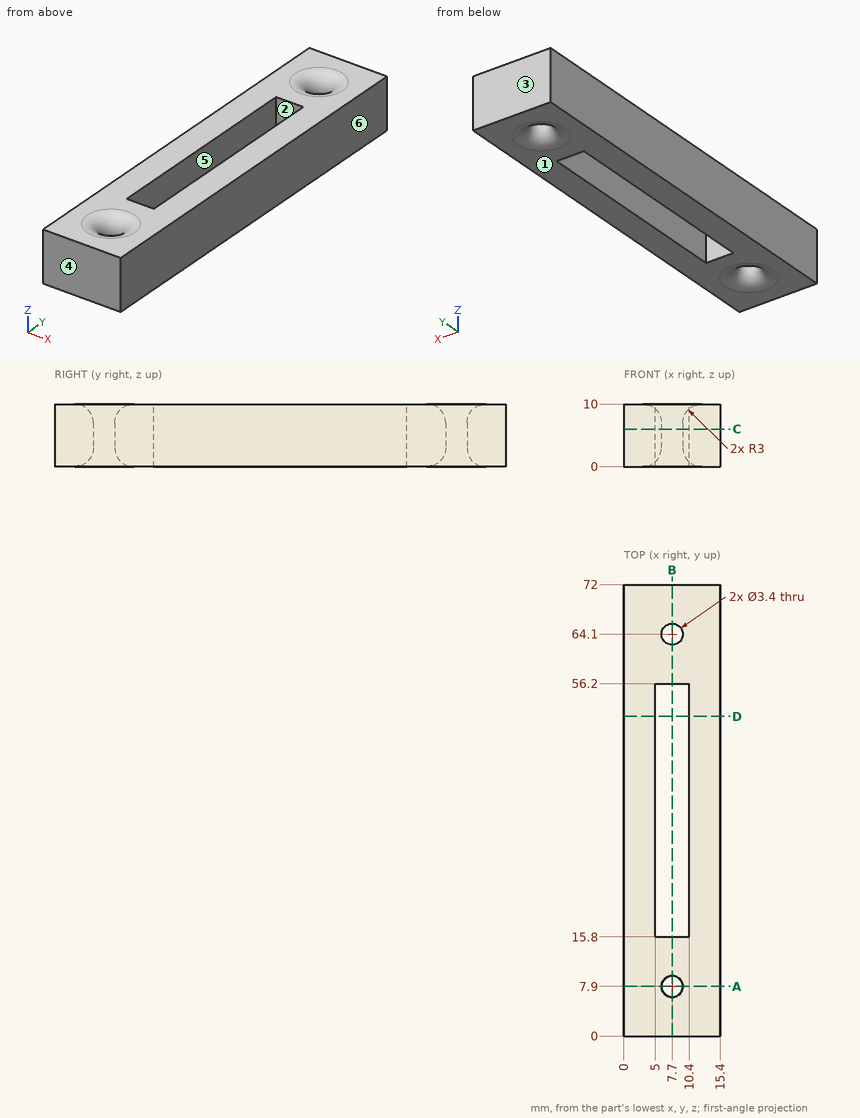
Design review of the part shown in the three views and the two pictorial views. Dimensions are in mm from the part's minimum x, y and z. A direction names the side the tool comes from. Give positions to 0.01 mm unless a question says otherwise; leave off trailing zeros. Loops run counter-clockwise (first coordinate to the right, second up) from the corner with the lowest first, then second, coordinate; pieces in that order, holes last. Notation, with made-up numbers: (67.25, -25) -> (102.25, -25) arc R16 ccw to (102.25, -1) -> close; hole circle Ø3 at (88, 71). An arc over 180 degrees is marked (long way). Answer as a JSON object with one key per item and string values. Group by question number.
Q1. Draft analysis for pull direction Y (two halves, no side actions). For the marked faces 1, 2, 3 and 4, state which applies: pulls with the +Y half, pulls with the -Y half, needs draft (parallel to the pull), parting line crosses it, or undercut.
Q2. Wall thickness on line 1 along Y through (x, z) = (7.7, 5.25); line 2 along X through (y, z) = (52, 7.25); line 3 along Y through (x, z) = (6.5, 1): over which ranges is each line inside the solid? List them lowest first.
Q3. Take a section at A-A (y = 7.9). Write out the cut boundary in (x, z), plus the area to 3 significant figures.
Q4. Take a section at C-C (z = 6). Write out the cut boundary in (x, y), plus the area to 3 significant figures.
Q5. Take a section at B-B (x = 7.7). Write out the cut boundary in (y, z).
Q6. Insertion check: pin 1 (4.5 mm diameter, centred on x = 7.7, y = 64.1, fed in from +Z); pin 2 (3 mm diameter, centred on x = 7.7, y = 7.9, fed in from -Z). Each pin has a flat end and moves straight along its axis. Give the tip position at first contact, or say it passes through.
Q7. Take a section at D-D (y = 51). Write out the cut boundary in (x, z).
Q8. Tool access review of the marked faces 5 and 6: name each direction out of +Z, -Z, +X, -X, +Y, -Y from which nothing blocks a thin tool from reaching the whole face with its end or side.
Answer below:
{
 "1": {"face 1": "needs draft", "face 2": "undercut", "face 3": "pulls with the +Y half", "face 4": "pulls with the -Y half"},
 "2": {"line 1": "y = 0 to 6.2, 9.6 to 15.8, 56.2 to 62.4, 65.8 to 72", "line 2": "x = 0 to 5, 10.4 to 15.4", "line 3": "y = 0 to 5.75, 10.05 to 15.8, 56.2 to 61.95, 66.25 to 72"},
 "3": {"outline": "(0, 0) -> (3, 0) arc R3 ccw to (6, 3) -> (6, 7) arc R3 ccw to (3, 10) -> (0, 10) -> close; (9.4, 3) arc R3 ccw to (12.4, 0) -> (15.4, 0) -> (15.4, 10) -> (12.4, 10) arc R3 ccw to (9.4, 7) -> close", "area": "112 mm2"},
 "4": {"outline": "(0, 0) -> (15.4, 0) -> (15.4, 72) -> (0, 72) -> close; hole (5, 15.8) -> (10.4, 15.8) -> (10.4, 56.2) -> (5, 56.2) -> close; hole circle Ø3.4 at (7.7, 7.9); hole circle Ø3.4 at (7.7, 64.1)", "area": "872 mm2"},
 "5": {"outline": "(0, 0) -> (3.2, 0) arc R3 ccw to (6.2, 3) -> (6.2, 7) arc R3 ccw to (3.2, 10) -> (0, 10) -> close; (9.6, 3) arc R3 ccw to (12.6, 0) -> (15.8, 0) -> (15.8, 10) -> (12.6, 10) arc R3 ccw to (9.6, 7) -> close; (56.2, 0) -> (59.4, 0) arc R3 ccw to (62.4, 3) -> (62.4, 7) arc R3 ccw to (59.4, 10) -> (56.2, 10) -> close; (65.8, 3) arc R3 ccw to (68.8, 0) -> (72, 0) -> (72, 10) -> (68.8, 10) arc R3 ccw to (65.8, 7) -> close"},
 "6": {"pin 1": "stops at z = 8.73", "pin 2": "passes through"},
 "7": {"outline": "(0, 0) -> (5, 0) -> (5, 10) -> (0, 10) -> close; (10.4, 0) -> (15.4, 0) -> (15.4, 10) -> (10.4, 10) -> close"},
 "8": {"face 5": "+Z, -Z", "face 6": "+Z, -Z, +X, +Y, -Y"}
}
